Geometry: final body of the model. Coordinates: model frame, mm. A direction names the side the tool comes from. Give positions to 0.01 mm unless a question says otherwise; leave off trailing zeros. Write each loop counter-clockwise with the first axis right and the second up, starting at its lowest first coordinate (ties: lowest second). Pieces come first, ordered by that corner, then holes. Notation, with made-up numbers: M 75,40.25 L 92,40.25 A32 cw 92,71.25 Z; hole C -22.75,39.5 d4. An arc over 180 degrees is marked long. Answer as a JSON object with one key per item and string values.
from build123d import *

# Parameters (mm, degrees)
F0_W          = 94.742008
F0_H          = 62.738002
F1_DEPTH      = 38.1
F2_R          = 16.414966
F3_DEPTH      = 25.4
F3_DEPTH_BACK = 12.7
F4_R          = 8.890001
F5_DEPTH      = 10.16


with BuildPart() as f1:
    # F0 (on Front) → F1 (new body)
    with BuildSketch(Plane.XZ):
        Rectangle(F0_W, F0_H)
    extrude(amount=F1_DEPTH)

    # F2 (on face) → F3 (join, two sides)
    with BuildSketch(Plane.XZ.offset(38.1)) as f3_sk:
        Circle(F2_R)
    extrude(amount=F3_DEPTH)
    extrude(f3_sk.sketch, amount=-F3_DEPTH_BACK)

    # F4 (on face) → F5 (join)
    with BuildSketch(Plane.XY.offset(31.369001)):
        with Locations((28.066998, -18.923)):
            Circle(F4_R)
    extrude(amount=F5_DEPTH)


solid = f1.part
1) Contact query for flat-ended pins moving along their axis: P1, Ø6, axis at y = -52, z = 12, coming from the +X side; P2, Ø10, axis at y = -48, z = 11, coming from the -X side; P3, Ø8, axis at y = -52.5, z = 7, coming from the +X side. Output: stop coordinate, or through.
Geometry check:
{"P1": "stops at x = 13.73", "P2": "stops at x = -15.28", "P3": "stops at x = 16.14"}
2) Line query: line 1 (Y direction, x = 26, z = -26); line 2 (Z direction, x = -12, y = -36); line 3 (X direction, y = -46.5, z = 12). Output: solid intervals per line, ascending. Write a range as from..to.
Geometry check:
{"line 1": "y = -38.1..0", "line 2": "z = -31.37..31.37", "line 3": "x = -11.2..11.2"}
3) Cut plane A-A on x = 0. Return loops of the section in (y, z), and give its area (3 significant figures).
Geometry check:
{"outline": "M -63.5,-16.41 L -38.1,-16.41 L -38.1,-31.37 L 0,-31.37 L 0,31.37 L -38.1,31.37 L -38.1,16.41 L -63.5,16.41 Z", "area": "3,220 mm2"}
4) Cut plane C-C on y = -31.5. Return loops of the section in (x, z), and give its area (3 significant figures).
Geometry check:
{"outline": "M -47.37,-31.37 L 47.37,-31.37 L 47.37,31.37 L -47.37,31.37 Z", "area": "5,940 mm2"}
5) Cut plane D-D on z = -21.5. Return loops of the section in (x, y), and give its area (3 significant figures).
Geometry check:
{"outline": "M -47.37,-38.1 L 47.37,-38.1 L 47.37,0 L -47.37,0 Z", "area": "3,610 mm2"}
6) Set-up query: faces 1 (the cylindrical face through (8.825, -50.622, 13.841)), 2 (the cylindrical face through (21.515, -12.915, 36.378)), 3 (the flat face through (28, -19, 41.529)). Return all of +Z, -Z, +X, -X, +Y, -Y with unobstructed straight access to the full face (end or side cutting, diameter ignored); none if empty.
Geometry check:
{"face 1": "-Y", "face 2": "+Z", "face 3": "+Z, +X, -X, +Y, -Y"}
7) Cut plane B-B on z = 0. Return loops of the section in (x, y), and give its area (3 significant figures).
Geometry check:
{"outline": "M -47.37,-38.1 L -16.41,-38.1 L -16.41,-63.5 L 16.41,-63.5 L 16.41,-38.1 L 47.37,-38.1 L 47.37,0 L -47.37,0 Z", "area": "4,440 mm2"}
